```python
from build123d import *

# Parameters (mm, degrees)
SKETCH1_R           = 5
BOSS_EXTRUDE1_DEPTH = 10


with BuildPart() as part:
    # Sketch1 → Boss-Extrude1 (new body)
    with BuildSketch(Plane.XY):
        Polygon((-15, 0), (15, 0), (15, 10), (25, 10), (25, 0), (35, 0), (35, 40), (25, 50), (-25, 50), (-35, 40), (-35, 0), (-25, 0), (-25, 10), (-15, 10), align=None)
        with Locations((25, 40)):
            Circle(SKETCH1_R, mode=Mode.SUBTRACT)
        with Locations((-25, 40)):
            Circle(SKETCH1_R, mode=Mode.SUBTRACT)
        Polygon((-5, 20), (5, 20), (5, 25), (15, 25), (15, 15), (-15, 15), (-15, 25), (-5, 25), align=None, mode=Mode.SUBTRACT)
    extrude(amount=BOSS_EXTRUDE1_DEPTH)


solid = part.part
```
The model under review builds one solid part; all positions refer to its coordinate system, in mm. A direction names the side the tool comes from. Round coordinates to 2 decimals unless told otherwise and drop trailing zeros. Loops run counter-clockwise (first coordinate to the right, second up) from the corner with the lowest first, then second, coordinate; pieces in that order, holes last.
1) Wall thickness on line 1 along X through (y, z) = (8.5, 8.75); line 2 along X through (y, z) = (39.5, 7); line 3 along X through (y, z) = (17, 7): over which ranges is each line inside the solid? List them lowest first.
Values follow:
line 1: x = -35 to -25, -15 to 15, 25 to 35
line 2: x = -35 to -29.97, -20.03 to 20.03, 29.97 to 35
line 3: x = -35 to -15, 15 to 35
2) Consider section D-D on y = 18. State the section outline as (x, z) points, then the cut area to 3 significant figures.
Values follow:
outline: (-35, 0) - (-15, 0) - (-15, 10) - (-35, 10) - close; (15, 0) - (35, 0) - (35, 10) - (15, 10) - close
area: 400 mm2
3) Consider section C-C on x = -21. State the section outline as (y, z) points.
Values follow:
outline: (10, 0) - (37, 0) - (37, 10) - (10, 10) - close; (43, 0) - (50, 0) - (50, 10) - (43, 10) - close
4) Consider section B-B on y = 7. State the section outline as (x, z) points, then the cut area to 3 significant figures.
Values follow:
outline: (-35, 0) - (-25, 0) - (-25, 10) - (-35, 10) - close; (-15, 0) - (15, 0) - (15, 10) - (-15, 10) - close; (25, 0) - (35, 0) - (35, 10) - (25, 10) - close
area: 500 mm2
5) The part is to be moulded in two halves that separate along X. For faces 4 (the face through (15, 20, 5)), 5 (the face through (0, 50, 5)), 6 (the face through (35, 20, 5)), say which applies: pulls with the +X half, pulls with the -X half, needs draft (parallel to the pull), parting line crosses it, or undercut.
Values follow:
face 4: undercut
face 5: needs draft
face 6: pulls with the +X half
6) Consider section A-A on z = 2.75. State the section outline as (x, y) points.
Values follow:
outline: (-35, 0) - (-25, 0) - (-25, 10) - (-15, 10) - (-15, 0) - (15, 0) - (15, 10) - (25, 10) - (25, 0) - (35, 0) - (35, 40) - (25, 50) - (-25, 50) - (-35, 40) - close; hole circle Ø10 at (-25, 40); hole (-15, 15) - (15, 15) - (15, 25) - (5, 25) - (5, 20) - (-5, 20) - (-5, 25) - (-15, 25) - close; hole circle Ø10 at (25, 40)
7) Tool access review of faces 1 (the face through (0, 25, 0)), 2 (the face through (-25, 5, 5)), 3 (the face through (5, 22, 5)): name each direction out of +Z, -Z, +X, -X, +Y, -Y from which nothing blocks a thin tool from reaching the whole face with its end or side.
Values follow:
face 1: -Z, +X, -X, +Y, -Y
face 2: +Z, -Z, -Y
face 3: +Z, -Z
